```python
from build123d import *

# Parameters (mm, degrees)
F0_W     = 101.6
F0_H     = 25.4
F1_DEPTH = 25.4
F2_R     = 3.96875
F3_DEPTH = 19.05
F4_R     = 3.96875
F5_DEPTH = 19.05


with BuildPart() as f1:
    # F0 (on Right) → F1 (new body)
    with BuildSketch(Plane.YZ):
        with Locations((50.8, 12.7)):
            Rectangle(F0_W, F0_H)
    extrude(amount=F1_DEPTH)

    # F2 (on face) → F3 (cut)
    with BuildSketch(Plane(origin=(0, 101.6, 0), x_dir=(-1, 0, 0), z_dir=(0, 1, 0))):
        with Locations((-12.7, 12.7)):
            Circle(F2_R)
    extrude(amount=-F3_DEPTH, mode=Mode.SUBTRACT)

    # F4 (on face) → F5 (cut)
    with BuildSketch(Plane.XZ):
        with Locations((13.019745, 12.7)):
            Circle(F4_R)
    extrude(amount=-F5_DEPTH, mode=Mode.SUBTRACT)


solid = f1.part
```
Check sheet for the modelled part. Datum: model origin and axes. Units: mm. A direction names the side the tool comes from. Give positions to 0.01 mm unless a question says otherwise; leave off trailing zeros. Loops run counter-clockwise (first coordinate to the right, second up) from the corner with the lowest first, then second, coordinate; pieces in that order, holes last. Notation, with made-up numbers: M 24.25,-4.5 L 34.25,-4.5 A20 ccw 34.25,24.5 Z; hole C 67,65 d4. An arc over 180 degrees is marked long. Answer in a Markdown table with one row per item.
1) Cross-section at B-B (x = 11.5). Enter the section's corners in (y, z), plus the area to 3 significant figures.
Solutions:
| item | result |
|---|---|
| outline | M 0,0 L 101.6,0 L 101.6,8.92 L 82.55,8.92 L 82.55,16.48 L 101.6,16.48 L 101.6,25.4 L 0,25.4 L 0,16.37 L 19.05,16.37 L 19.05,9.03 L 0,9.03 Z |
| area | 2,300 mm^2 |
2) Thickness scan on line 1 (Z direction, x = 12.7, y = 95.25); line 2 (Z direction, x = 12, y = 17); line 3 (Y direction, x = 12.5, z = 14). Record the ranges inside material, lowest first.
Solutions:
| item | result |
|---|---|
| line 1 | z = 0 to 8.73, 16.67 to 25.4 |
| line 2 | z = 0 to 8.86, 16.54 to 25.4 |
| line 3 | y = 19.05 to 82.55 |
3) Mould release check, pull along X, two halves, no side actions. Record for faces 3 (the face through (13, 82.55, 13)), 4 (the face through (9.034, 92.208, 11.18)), 5 (the face through (0, 50, 13)), 6 (the face through (13, 50, 25.4)): released by +X, released by -X, zero draft, split by the parting line, or undercut.
Solutions:
| item | result |
|---|---|
| face 3 | undercut |
| face 4 | undercut |
| face 5 | released by -X |
| face 6 | zero draft |
4) Depth check by flat-ended pin: pin 1 (4 mm diameter, centred on x = 13.5, z = 14, fed in from -Y). Enter the tip coordinate at first touch or a pass-through.
Solutions:
| item | result |
|---|---|
| pin 1 | stops at y = 19.05 |
5) Tool access check on faces 1 (the face through (12.159, 9.392, 8.826)), 2 (the face through (9.7, 0, 15.3)). Record the directions out of +Z, -Z, +X, -X, +Y, -Y that give a thin tool (end or side, any length) a straight path to the whole face; none if there is none.
Solutions:
| item | result |
|---|---|
| face 1 | -Y |
| face 2 | +Z, -Z, +X, -X, -Y |
6) Cross-section at A-A (z = 12.7). Enter the section's corners in (x, y), plus the area to 3 significant figures.
Solutions:
| item | result |
|---|---|
| outline | M 0,0 L 9.05,0 L 9.05,19.05 L 16.99,19.05 L 16.99,0 L 25.4,0 L 25.4,101.6 L 16.67,101.6 L 16.67,82.55 L 8.73,82.55 L 8.73,101.6 L 0,101.6 Z |
| area | 2,280 mm^2 |
